Source: CAD feature listing. Evaluate the final solid. Frame: model axes, mm. Face numbers are marked on the shaded views. A direction names the side the tool comes from. Give positions to 0.01 mm unless a question says otherwise; leave off trailing zeros. Order: outer loops, then holes, each group sorted by start corner. A loop starts at its lowest first (then second) coordinate and runs counter-clockwise, first axis right, second up. Notation, with made-up numbers: (56, -28) - (64, -28) arc R18 ccw to (64, 3) - close; hole circle Ø7 at (51.5, 72). An arc over 180 degrees is marked (long way). One line per item, written item: value. Start each with the question number.
Autodesk Inventor part; units mm, degrees
ref_plane "YZ Plane" through (0, 0, 0) normal (1, 0, 0) x (0, 1, 0)
ref_plane "XZ Plane" through (0, 0, 0) normal (0, 1, 0) x (-1, 0, 0)
ref_plane "XY Plane" through (0, 0, 0) normal (0, 0, 1) x (1, 0, 0)
sketch "Sketch1" plane through (0, 0, 0) normal (0, 1, 0) x (-1, 0, 0)
  line L0 (0, 0) -> (27.94, 0)
  line L1 (27.94, 0) -> (27.94, -53.34)
  line L2 (27.94, -53.34) -> (0, -53.34)
  line L3 (0, -53.34) -> (0, 0)
  dimension "d0" = 27.94
  dimension "d1" = 53.34
extrude "Extrusion1" add sketch "Sketch1" along normal blind 15.24
shell "Shell1" thickness 2.54 removed faces 1 at (-9.3133, 15.24, -17.78)
sketch "Sketch3" plane through (-27.94, 0, 0) normal (0, 0, 1) x (1, 0, 0)
  line L0 (20.32, 5.08) -> (7.62, 5.08)
  line L1 (7.62, 5.08) -> (7.62, 10.16)
  line L2 (7.62, 10.16) -> (20.32, 10.16)
  line L3 (20.32, 10.16) -> (20.32, 5.08)
  point P0 (27.94, 0)
  dimension "d20" = 5.08
  dimension "d21" = 12.7
  dimension "d22" = 5.08
  dimension "d23" = 7.62
extrude "Extrusion3" cut sketch "Sketch3" against normal blind 2.54
chamfer "Chamfer1" distance 3.175 angle 45 2 edges at (-20.32, 10.16, -1.27) (-7.62, 10.16, -1.27)
sketch "Sketch5" plane through (-25.4, 2.54, -2.54) normal (0, 1, 0) x (1, 0, 0)
  line L0 (0, 0) -> (5.334, 0)
  line L1 (5.334, 0) -> (5.334, 48.26)
  line L2 (5.334, 48.26) -> (0, 48.26)
  line L3 (0, 48.26) -> (0, 0)
  line L4 (0, 48.26) -> (22.86, 48.26)
  line L5 (22.86, 0) -> (17.526, 0)
  line L6 (17.526, 0) -> (17.526, 48.26)
  line L7 (17.526, 48.26) -> (22.86, 48.26)
  line L8 (22.86, 48.26) -> (22.86, 0)
  point P0 (25.4, -2.54)
  dimension "d29" = 5.334
  dimension "d30" = 5.334
extrude "Extrusion4" cut sketch "Sketch5" against normal blind 2.54
sketch "Sketch6" plane through (-27.94, 0, -53.34) normal (-1, 0, 0) x (0, 0, 1)
  point P0 (53.34, 0)
sketch "Sketch7" plane through (-27.94, 0, -53.34) normal (-1, 0, 0) x (0, 0, 1)
  line L0 (2.54, 15.24) -> (50.8, 15.24)
  line L1 (0, 0) -> (2.54, 0)
  line L2 (2.54, 0) -> (2.54, 15.24)
  line L3 (2.54, 15.24) -> (0, 15.24)
  line L4 (0, 15.24) -> (0, 0)
  point P0 (53.34, 0)
  dimension "d33" = 2.54
extrude "Extrusion5" add sketch "Sketch7" along normal blind 5.08
sketch "Sketch8" plane through (-27.94, 0, -50.8) normal (0, 0, 1) x (1, 0, 0)
  line L0 (-5.08, 15.24) -> (-2.54, 15.24)
  line L1 (-2.54, 15.24) -> (-2.54, 0)
  line L2 (-2.54, 0) -> (-5.08, 0)
  line L3 (-5.08, 0) -> (-5.08, 15.24)
  point P0 (27.94, 0)
  dimension "d36" = 2.54
extrude "Extrusion6" add sketch "Sketch8" along normal up to surface (50.8 mm away)
chamfer "Chamfer2" distance 1.27 angle 45 6 edges at (-2.54, 0, -26.67) (-5.207, 0, -2.54) (-5.207, 0, -50.8) (-22.733, 0, -2.54) (-25.4, 0, -26.67) (-22.733, 0, -50.8)
sketch "Sketch11" plane through (0, 15.24, 0) normal (0, 1, 0) x (1, 0, 0)
  line L0 (-26.67, 52.07) -> (-17.78, 52.07)
  line L1 (-20.32, 1.27) -> (-26.67, 1.27)
  line L2 (-26.67, 1.27) -> (-26.67, 52.07)
  line L3 (-25.4, 2.54) -> (-25.4, 50.8)
  line L4 (-2.54, 2.54) -> (-25.4, 2.54)
  line L5 (-25.4, 50.8) -> (-2.54, 50.8)
  line L6 (-1.27, 52.07) -> (-7.62, 52.07)
  line L7 (-7.874, 1.27) -> (-1.27, 1.27)
  line L8 (-1.27, 1.27) -> (-1.27, 52.07)
  line L9 (-2.54, 50.8) -> (-2.54, 2.54)
  line L10 (-7.62, 52.07) -> (-1.27, 52.07)
  line L11 (-1.27, 52.07) -> (-1.27, 50.8)
  line L12 (-1.27, 50.8) -> (-7.62, 50.8)
  line L13 (-7.62, 50.8) -> (-7.62, 52.07)
  line L14 (-2.54, 50.8) -> (-1.27, 50.8)
  line L15 (-1.27, 50.8) -> (-1.27, 1.27)
  line L16 (-1.27, 1.27) -> (-2.54, 1.27)
  line L17 (-2.54, 1.27) -> (-2.54, 50.8)
  line L18 (-2.54, 2.54) -> (-7.874, 2.54)
  line L19 (-7.874, 2.54) -> (-7.874, 1.27)
  line L20 (-7.874, 1.27) -> (-2.54, 1.27)
  line L21 (-2.54, 1.27) -> (-2.54, 2.54)
  line L22 (-26.67, 52.07) -> (-20.32, 52.07)
  line L23 (-20.32, 52.07) -> (-20.32, 50.8)
  line L24 (-20.32, 50.8) -> (-26.67, 50.8)
  line L25 (-26.67, 50.8) -> (-26.67, 52.07)
  line L26 (-25.4, 50.8) -> (-26.67, 50.8)
  line L27 (-26.67, 50.8) -> (-26.67, 1.27)
  line L28 (-26.67, 1.27) -> (-25.4, 1.27)
  line L29 (-25.4, 1.27) -> (-25.4, 50.8)
  line L30 (-25.4, 2.54) -> (-20.32, 2.54)
  line L31 (-20.32, 2.54) -> (-20.32, 1.27)
  line L32 (-20.32, 1.27) -> (-25.4, 1.27)
  line L33 (-25.4, 1.27) -> (-25.4, 2.54)
  point P0 (0, 0)
  dimension "d50" = 1.27
  dimension "d51" = 1.27
  dimension "d52" = 1.27
  dimension "d55" = 1.27
  dimension "d57" = 1.27
  dimension "d58" = 5.08
  dimension "d59" = 48.26
  dimension "d60" = 6.35
  dimension "d61" = 6.35
extrude "Extrusion8" add sketch "Sketch11" along normal blind 1.27 contours L0 L23 L5 L24 L2 | L24 L3 L29 L1 L2 | L13 L6 L8 L12 L5 | L29 L4 L31 L1 | L12 L8 L7 L17 L9 | L17 L7 L19 L4
chamfer "Chamfer3" distance 1.27 angle 45 6 edges at (-1.27, 16.51, -26.67) (-4.572, 16.51, -1.27) (-4.445, 16.51, -52.07) (-23.495, 16.51, -52.07) (-26.67, 16.51, -26.67) (-23.495, 16.51, -1.27)
sketch "Sketch12" plane through (0, 0, 0) normal (1, 0, 0) x (0, 0, -1)
  line L0 (52.07, 0) -> (1.27, 0)
  line L1 (0, 15.24) -> (53.34, 15.24)
  line L2 (19.05, 0) -> (34.29, 0)
  line L3 (34.29, 0) -> (34.29, 15.24)
  line L4 (34.29, 15.24) -> (19.05, 15.24)
  line L5 (19.05, 15.24) -> (19.05, 0)
  line L6 (0, 0) -> (0, 15.24)
  line L7 (53.34, 0) -> (53.34, 15.24)
  dimension "d67" = 19.05
  dimension "d68" = 19.05
extrude "Extrusion9" add sketch "Sketch12" along normal blind 2.54
sketch "Sketch14" plane through (0, 0, 0) normal (0, -1, 0) x (1, 0, 0)
  line L0 (0, -19.05) -> (0, -21.59)
  line L1 (2.54, -19.05) -> (0, -21.59)
  line L2 (0, -34.29) -> (0, -31.75)
  line L3 (0, -31.75) -> (2.54, -34.29)
  line L4 (0, -19.05) -> (2.54, -19.05)
  line L5 (0, -19.05) -> (2.54, -19.05)
  line L6 (2.54, -34.29) -> (0, -34.29)
  line L7 (0, -53.34) -> (0, -34.29)
  point P0 (0, 0)
  dimension "d71" = 2.54
  dimension "d72" = 2.54
extrude "Extrusion10" cut sketch "Sketch14" against normal blind 25.4
properties part number "nano_enclosure_modular"
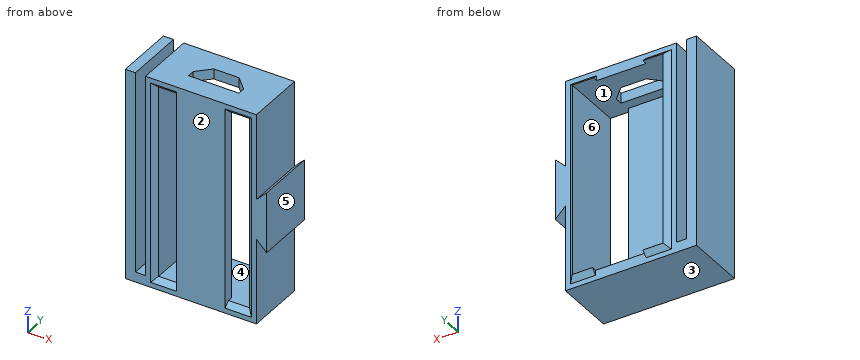
1. Set-up query: the marked faces 4, 5 and 6. Return all of +Z, -Z, +X, -X, +Y, -Y with unobstructed straight access to the full face (end or side cutting, diameter ignored); none if empty.
2. Ray query, L1, parallel to X at y = 14, z = -16; L2, parallel to X at y = 12, z = -24; L3, parallel to X at y = 2, z = -16.5. Return the intervals inside material, ascending.
3. Draft query along Z for the marked faces 1, 2 and 3. Return one class per face: pulls with the +Z half, pulls with the -Z half, needs draft (parallel to the pull), parting line crosses it, or undercut.
4. Section D-D on x = -10. Return the cut outline in (y, z) (3 decimals).
5. Section C-C on y = 4.5. Return the cut outline in (x, z), then the cut area to 3 significant figures.
6. Section A-A on z = -35.5. Count the separate pieces of the cut face and the enclosed holes in it, then the cut area to 3 significant figures.
7. Contact query for flat-ended pins moving along their axis: pin 1 Ø7.5 at (y, z) = (6.5, -15) entering from +X; pin 2 Ø1.3 at (x, y) = (-29.5, 8) entering from +Z; pin 3 Ø1.4 at (y, z) = (16, -2) entering from -X. Output: stop coordinate, or through.
Data:
1. face 4: +Y
1. face 5: +Z, -Z, +X, +Y, -Y
1. face 6: +Y, -Y
2. L1: x = -33.02 to -30.48, -27.94 to -25.4, -2.54 to 0
2. L2: x = -33.02 to -30.48, -27.94 to -25.4, -2.54 to 2.54
2. L3: x = -33.02 to -30.48, -27.94 to -25.4, -20.07 to -7.87, -2.54 to 0
3. face 1: undercut
3. face 2: needs draft
3. face 3: pulls with the -Z half
4. outline: (0, -53.34) - (15.24, -53.34) - (15.24, -50.8) - (2.54, -50.8) - (2.54, -2.54) - (5.08, -2.54) - (5.08, 0) - (0, 0) - close; (9.365, -2.54) - (15.24, -2.54) - (15.24, 0) - (9.365, 0) - close
5. outline: (-33.02, -53.34) - (0, -53.34) - (0, -31.75) - (2.54, -34.29) - (2.54, -19.05) - (0, -21.59) - (0, 0) - (-27.94, 0) - (-27.94, -50.8) - (-30.48, -50.8) - (-30.48, 0) - (-33.02, 0) - close; hole (-25.4, -50.8) - (-2.54, -50.8) - (-2.54, -2.54) - (-25.4, -2.54) - close
5. area: 561 mm2
6. separate pieces: 4
6. enclosed holes: 0
6. area: 147 mm2
7. pin 1: stops at x = 0
7. pin 2: stops at z = -50.8
7. pin 3: stops at x = -26.61
